from build123d import *

# Parameters (mm, degrees)
ESQUISSE1_R              = 47.75
BOSS_EXTRU_1_DEPTH       = 50
ESQUISSE2_R              = 26
ENL_V_MAT_EXTRU_1_DEPTH  = 20
ESQUISSE3_R              = 11
ENL_V_MAT_EXTRU_5_DEPTH  = 7.5
ESQUISSE4_R              = 5
ENL_V_MAT_EXTRU_6_DEPTH  = 13.5
ESQUISSE11_R             = 2.75
ENL_V_MAT_EXTRU_11_DEPTH = 85.024549984


with BuildPart() as part:
    # Esquisse1 → Boss.-Extru.1 (new body)
    with BuildSketch(Plane(origin=(0, 0, 0), x_dir=(1, 0, 0), z_dir=(0, 1, 0))):
        with Locations(Location((0, 0, 0), (0, 0, 270))):
            Circle(ESQUISSE1_R)
    extrude(amount=BOSS_EXTRU_1_DEPTH)

    # Esquisse2 → Enlèv. mat.-Extru.1 (cut)
    with BuildSketch(Plane(origin=(0, 0, 0), x_dir=(-1, 0, 0), z_dir=(0, -1, 0))):
        with Locations(Location((0, 0, 0), (0, 0, 90))):
            Circle(ESQUISSE2_R)
    extrude(amount=-ENL_V_MAT_EXTRU_1_DEPTH, mode=Mode.SUBTRACT)

    # Esquisse3 → Enlèv. mat.-Extru.5 (cut)
    with BuildSketch(Plane(origin=(0, 20, 0), x_dir=(-1, 0, 0), z_dir=(0, -1, 0))):
        with Locations(Location((0, 0, 0), (0, 0, 90))):
            Circle(ESQUISSE3_R)
    extrude(amount=-ENL_V_MAT_EXTRU_5_DEPTH, mode=Mode.SUBTRACT)

    # Esquisse4 → Enlèv. mat.-Extru.6 (cut)
    with BuildSketch(Plane(origin=(0, 27.5, 0), x_dir=(-1, 0, 0), z_dir=(0, -1, 0))):
        with Locations(Location((0, 0, 0), (0, 0, 90))):
            Circle(ESQUISSE4_R)
    extrude(amount=-ENL_V_MAT_EXTRU_6_DEPTH, mode=Mode.SUBTRACT)

    # Esquisse11 → Enlèv. mat.-Extru.11 (cut, through all)
    with BuildSketch(Plane(origin=(0, 50, 0), x_dir=(1, 0, 0), z_dir=(0, 1, 0))):
        with Locations(Location((-16, 0, 0), (0, 0, 270))):
            Circle(ESQUISSE11_R)
        with Locations(Location((0, 16, 0), (0, 0, 270))):
            Circle(ESQUISSE11_R)
        with Locations(Location((16, 0, 0), (0, 0, 270))):
            Circle(ESQUISSE11_R)
        with Locations(Location((0, -16, 0), (0, 0, 270))):
            Circle(ESQUISSE11_R)
    extrude(amount=-ENL_V_MAT_EXTRU_11_DEPTH, mode=Mode.SUBTRACT)


solid = part.part
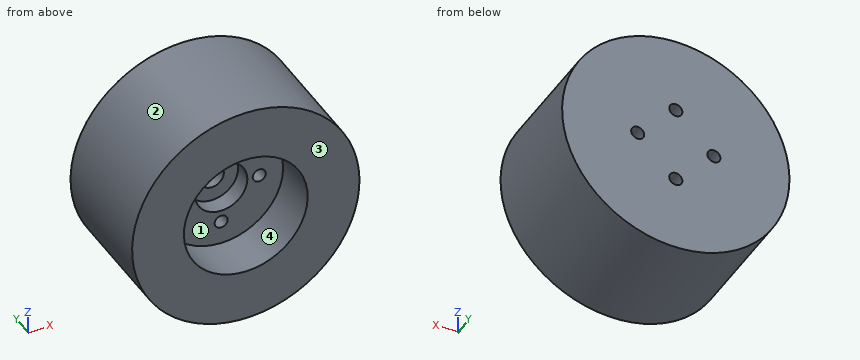
Could you check a few things on this model? Use its own coordinates, in mm. Face numbers are marked on the shaded views. Round coordinates to 2 decimals unless told otherwise and drop trailing zeros. Write each loop counter-clockwise with the first axis right and the second up, starting at its lowest first coordinate (ties: lowest second). Pieces come first, ordered by that corner, then holes. Notation, with made-up numbers: (87, 83.25) - (146, 83.25) arc R20 cw to (146, 120.25) - close; hole circle Ø5 at (14.25, -30). An arc over 180 degrees is marked (long way). Put each result on its own line as item: value. Start each with the question number.
(1) I want a section at C-C, the plane y = 31.5. Please give me the cut outline in (x, z).
(2) I want a section at D-D, the plane x = 16. Please give me the cut outline in (y, z).
(3) Thinking about a two-plate mould opening in Z: for the marked faces 1, 2, 3 and 4, which applies, released by +Z, released by -Z, zero draft, split by the parting line, or undercut?
(4) Will these pins go through, and if not, where does the flat tip stop? pin 1 (9 mm diameter, centred on x = 0, z = 0, fed in from -Y); pin 2 (3.5 mm diameter, centred on x = 16, z = 0, fed in from -Y); pin 3 (17.5 mm diameter, centred on x = -0.5, z = -4, fed in from -Y); pin 4 (3 mm diameter, centred on x = 3, y = 28, fed in from -Z).
(5) I want a section at B-B, the plane x = 0. Please give me the cut outline in (y, z), plus the area to 4 significant figures.
(6) I need wall thicknesses on probe 1 along X at (y, z) = (23, 0); probe 2 along Z at (x, y) = (-1.5, 36); probe 3 along Z at (x, y) = (14, 10). Which ranges of each line are inside material? Lowest first, please.
(7) I want a section at A-A, the plane z = 0. Please give me the cut outline in (x, y).
Here are the results:
1. outline: circle Ø95.5 at (0, 0); hole circle Ø5.5 at (-16, 0); hole circle Ø10 at (0, 0); hole circle Ø5.5 at (0, -16); hole circle Ø5.5 at (0, 16); hole circle Ø5.5 at (16, 0)
2. outline: (0, -44.99) - (50, -44.99) - (50, -2.75) - (20, -2.75) - (20, -20.49) - (0, -20.49) - close; (0, 20.49) - (20, 20.49) - (20, 2.75) - (50, 2.75) - (50, 44.99) - (0, 44.99) - close
3. face 1: undercut
3. face 2: split by the parting line
3. face 3: zero draft
3. face 4: undercut
4. pin 1: stops at y = 41
4. pin 2: passes through
4. pin 3: stops at y = 20
4. pin 4: stops at z = -47.73
5. outline: (0, -47.75) - (50, -47.75) - (50, -18.75) - (20, -18.75) - (20, -26) - (0, -26) - close; (0, 26) - (20, 26) - (20, 18.75) - (50, 18.75) - (50, 47.75) - (0, 47.75) - close; (20, -13.25) - (50, -13.25) - (50, 13.25) - (20, 13.25) - (20, 11) - (27.5, 11) - (27.5, 5) - (41, 5) - (41, -5) - (27.5, -5) - (27.5, -11) - (20, -11) - close
5. area: 3,105 mm^2
6. probe 1: x = -47.75 to -18.75, -13.25 to -11, 11 to 13.25, 18.75 to 47.75
6. probe 2: z = -47.73 to -18.3, -13.7 to -4.77, 4.77 to 13.7, 18.3 to 47.73
6. probe 3: z = -45.65 to -21.91, 21.91 to 45.65
7. outline: (-47.75, 0) - (-26, 0) - (-26, 20) - (-18.75, 20) - (-18.75, 50) - (-47.75, 50) - close; (-13.25, 20) - (-11, 20) - (-11, 27.5) - (-5, 27.5) - (-5, 41) - (5, 41) - (5, 27.5) - (11, 27.5) - (11, 20) - (13.25, 20) - (13.25, 50) - (-13.25, 50) - close; (18.75, 20) - (26, 20) - (26, 0) - (47.75, 0) - (47.75, 50) - (18.75, 50) - close
